Geometry check sheet. Reference: the model listing, model coordinates, mm. Face numbers are marked on the shaded views. A direction names the side the tool comes from. Coordinates: 2 decimals unless noted, no trailing zeros. Order: outer loops, then holes, each group sorted by start corner. A loop starts at its lowest first (then second) coordinate and runs counter-clockwise, first axis right, second up. Notation, with made-up numbers: M 81.5,32.25 L 118.5,32.25 A27 ccw 118.5,66.25 Z; hole C 20.5,54.25 d1. An arc over 180 degrees is marked long. One line per item, written item: value. Start each with the question number.
1) Access from +Z, -Z, +X, -X, +Y, -Y to the whole of each face (thin tool, end or side, straight path). Record for the marked faces 5, 6 and 7.
2) Sectioned sample at B-B, the plane z = 75.5. Enter the section's corners in (x, y), then the cut area to 3 significant figures.
3) Sectioned sample at A-A, the plane y = 37.5. Enter the section's corners in (x, z).
4) Thickness scan on L1, parallel to Z at x = 33, y = 37; L2, parallel to Y at x = 24, z = 3; L3, parallel to Z at x = 42.5, y = 73. Record the ranges inside material, lowest first. Write a range as from..to.
5) Go/stop test with flat-tipped pins: P1, Ø5, axis at x = 18.5, z = 75, coming from the +Y side; P2, Ø10, axis at x = 34, z = 69.5, coming from the -Y side; P3, Ø8, axis at x = 16.5, y = 46, coming from the +Z side. Record where each tip stops, or that it passes through.
6) Draft check along Z on the marked faces 1, 2, 3 and 4. Enter one of: pulls with the +Z half, pulls with the -Z half, needs draft (parallel to the pull), parting line crosses it, or undercut.
```python
from build123d import *

# Parameters (mm, degrees)
F1_DEPTH = 59.967
F2_DEPTH = 16.11587
F3_DEPTH = 18.27724
F4_DEPTH = 18.65924
F5_DEPTH = 20.01095


with BuildPart() as f1:
    # F0 (on Right) → F1 (new body)
    with BuildSketch(Plane.YZ):
        Polygon((19.3016365517, 25.5114351168), (34.1311297964, 14.8414346621), (52.4001107586, 14.9257803925), (67.1304496505, 25.7322551057), (72.6956576812, 43.1331527599), (66.9700145375, 60.481921886), (52.1405212928, 71.1519223406), (33.8715403306, 71.0675766103), (30.248601096, 68.4097150693), (34.5660174948, 55.3278902953), (19.2159686951, 44.0667838525), (14.944761002, 47.1399696503), (13.575993408, 42.8602042428), align=None)
        Polygon((43.3843278169, 42.5439793365), (43.2058611327, 42.8390985452), (43.0657899565, 43.1542584575), (42.9663232941, 43.4844888132), (42.9090297944, 43.8245816823), (42.8948130101, 44.1691735971), (42.9238971483, 44.5128301373), (42.9958235348, 44.850131634), (43.1094578475, 45.175758641), (43.2630080055, 45.484575826), (43.454052431, 45.7717129574), (43.6795782392, 46.0326417111), (43.9360287536, 46.2632470849), (44.2193595962, 46.4598922942), (44.5251024704, 46.6194761267), (44.8484356285, 46.7394818499), (45.1842599134, 46.8180169019), (45.5272791756, 46.853842738), (45.8720837963, 46.8463943634), (46.2132360006, 46.7957892434), (46.5453556147, 46.7028254509), (46.8632049136, 46.5689690806), (47.1617712242, 46.3963311273), (47.4363459773, 46.1876341948), (47.6825989651, 45.9461695581), (47.8966466309, 45.6757452591), (48.075113315, 45.3806260503), (48.2151844913, 45.065466138), (48.3146511536, 44.7352357824), (48.3719446533, 44.3951429133), (48.3861614376, 44.0505509984), (48.3570772994, 43.7068944582), (48.2851509129, 43.3695929615), (48.1715166002, 43.0439659545), (48.0179664422, 42.7351487696), (47.8269220168, 42.4480116382), (47.6013962085, 42.1870828844), (47.3449456942, 41.9564775106), (47.0616148515, 41.7598323013), (46.7558719773, 41.6002484689), (46.4325388192, 41.4802427457), (46.0967145343, 41.4017076937), (45.7536952721, 41.3658818576), (45.4088906515, 41.3733302322), (45.0677384471, 41.4239353522), (44.7356188331, 41.5168991446), (44.4177695341, 41.6507555149), (44.1192032235, 41.8233934682), (43.8446284704, 42.0320904008), (43.5983754826, 42.2735550374), align=None, mode=Mode.SUBTRACT)
    extrude(amount=F1_DEPTH)

    # F2 (add): a face of the model
    f2_faces = [f1.faces().sort_by_distance(p)[0] for p in [
        (29.9835, 43.0060308117, 71.1097494755),
    ]]
    extrude(f2_faces, amount=F2_DEPTH)

    # F3 (add): a face of the model
    f3_faces = [f1.faces().sort_by_distance(p)[0] for p in [
        (29.9835, 69.8328361093, 51.8075373229),
    ]]
    extrude(f3_faces, amount=F3_DEPTH)

    # F4 (add): a face of the model
    f4_faces = [f1.faces().sort_by_distance(p)[0] for p in [
        (29.9835, 59.7652802045, 20.3290177491),
    ]]
    extrude(f4_faces, amount=F4_DEPTH)

    # F5 (add): a face of the model
    f5_faces = [f1.faces().sort_by_distance(p)[0] for p in [
        (29.9835, 26.7163831741, 20.1764348894),
    ]]
    extrude(f5_faces, amount=F5_DEPTH)


solid = f1.part
```
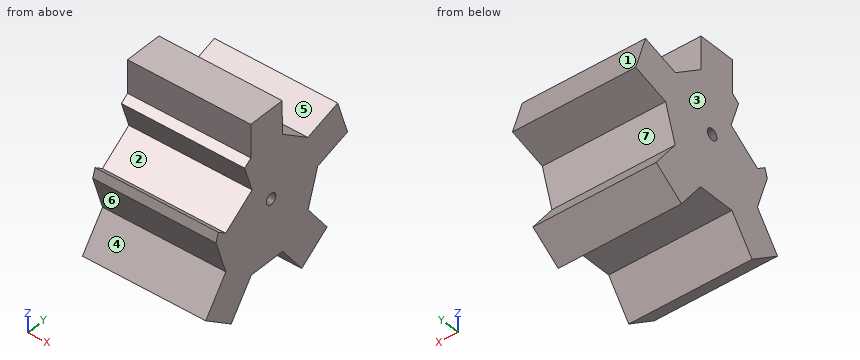
Final values:
1. face 5: +Z, +X, -X
1. face 6: +X, -X, -Y
1. face 7: +X, -X, +Y
2. outline: M 0,33.85 L 59.97,33.85 L 59.97,52.12 L 0,52.12 Z
2. area: 1,100 mm^2
3. outline: M 0,14.86 L 59.97,14.86 L 59.97,87.2 L 0,87.2 Z
4. L1: z = 14.85..87.2
4. L2: y = 16.33..25.61, 61.15..67.69
4. L3: z = 6.9..17.73, 43.23..62.47
5. P1: stops at y = 52.13
5. P2: stops at y = 30.25
5. P3: stops at z = 87.26
6. face 1: pulls with the +Z half
6. face 2: undercut
6. face 3: needs draft
6. face 4: undercut
